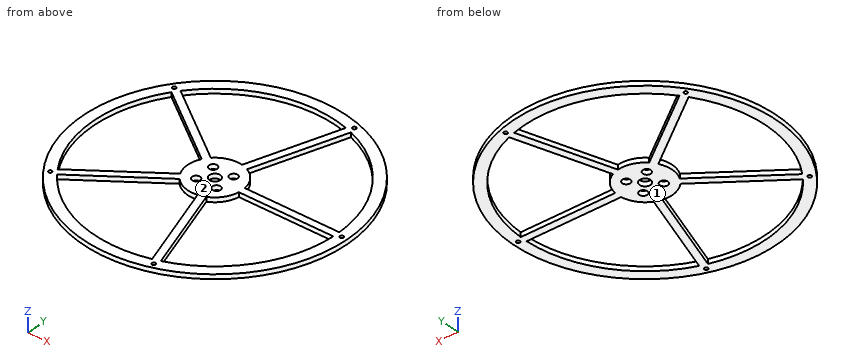
```python
from build123d import *

# Parameters (mm, degrees)
SKETCH_3_R          = 73
EXTRUDE_3_DEPTH     = 2.5
SKETCH_5_R          = 67
CUT_EXTRUDE_1_DEPTH = 2.5
SKETCH_6_R          = 15
EXTRUDE_4_DEPTH     = 2.5
SKETCH_7_R          = 8
CUT_EXTRUDE_2_DEPTH = 2.5
EXTRUDE_6_DEPTH     = 2.5
EXTRUDE_7_DEPTH     = 2.5
EXTRUDE_8_DEPTH     = 2.5
EXTRUDE_9_DEPTH     = 2.5
EXTRUDE_10_DEPTH    = 2.5
SKETCH_14_R         = 8
CUT_EXTRUDE_3_DEPTH = 2.5
SKETCH_15_R         = 1
CUT_EXTRUDE_4_DEPTH = 2.5
SKETCH_16_R         = 8
EXTRUDE_11_DEPTH    = 2.5
SKETCH_17_R         = 3
CUT_EXTRUDE_5_DEPTH = 2.5
SKETCH_18_R         = 3.25
SKETCH_18_R_2       = 2.2
CUT_EXTRUDE_6_DEPTH = 2.5
SKETCH_19_R         = 3.25
EXTRUDE_12_DEPTH    = 2.5
SKETCH_20_R         = 2.2
CUT_EXTRUDE_7_DEPTH = 2.5


with BuildPart() as part:
    # Sketch 3 → Extrude 3 (new body)
    with BuildSketch(Plane.XY):
        Circle(SKETCH_3_R)
    extrude(amount=EXTRUDE_3_DEPTH)

    # Sketch 5 → Cut-Extrude 1 (cut)
    with BuildSketch(Plane.XY.offset(2.5)):
        Circle(SKETCH_5_R)
    extrude(amount=-CUT_EXTRUDE_1_DEPTH, mode=Mode.SUBTRACT)



with BuildPart() as body_2:
    # Sketch 6 → Extrude 4 (new body)
    with BuildSketch(Plane.XY.offset(2.5)):
        Circle(SKETCH_6_R)
    extrude(amount=-EXTRUDE_4_DEPTH)

    # Sketch 7 → Cut-Extrude 2 (cut)
    with BuildSketch(Plane.XY.offset(2.5)):
        Circle(SKETCH_7_R)
    extrude(amount=-CUT_EXTRUDE_2_DEPTH, mode=Mode.SUBTRACT)


with BuildPart() as part_1:
    add(part.part)

    add(body_2.part)  # Extrude 6 merges body 2
    # Sketch 9 → Extrude 6 (add)
    with BuildSketch(Plane.XY.offset(2.5)):
        with BuildLine():
            Line((0, 2), (0, 0))
            Line((0, 0), (0, -2))
            Line((0, -2), (66.970142601, -2))
            ThreePointArc((66.970142601, -2), (67, 0), (66.970142601, 2))
            Line((66.970142601, 2), (0, 2))
        make_face()
    extrude(amount=-EXTRUDE_6_DEPTH)

    # Sketch 10 → Extrude 7 (add)
    with BuildSketch(Plane.XY.offset(2.5)):
        with BuildLine():
            Line((1.902113033, -0.618033989), (0, 0))
            Line((0, 0), (-1.902113033, 0.618033989))
            Line((-1.902113033, 0.618033989), (18.792799147, 64.310424507))
            ThreePointArc((18.792799147, 64.310424507), (20.704138623, 63.720786592), (22.597025212, 63.074356529))
            Line((22.597025212, 63.074356529), (1.902113033, -0.618033989))
        make_face()
    extrude(amount=-EXTRUDE_7_DEPTH)

    # Sketch 11 → Extrude 8 (add)
    with BuildSketch(Plane.XY.offset(2.5)):
        with BuildLine():
            Line((0, 0), (1.175570505, 1.618033989))
            Line((1.175570505, 1.618033989), (-53.004412975, 40.982096154))
            ThreePointArc((-53.004412975, 40.982096154), (-54.204138623, 39.381611904), (-55.355553985, 37.746028176))
            Line((-55.355553985, 37.746028176), (-1.175570505, -1.618033989))
            Line((-1.175570505, -1.618033989), (0, 0))
        make_face()
    extrude(amount=-EXTRUDE_8_DEPTH)

    # Sketch 12 → Extrude 9 (add)
    with BuildSketch(Plane.XY.offset(2.5)):
        with BuildLine():
            Line((0, 0), (1.175570505, -1.618033989))
            Line((1.175570505, -1.618033989), (-53.004412975, -40.982096154))
            ThreePointArc((-53.004412975, -40.982096154), (-54.176759621, -39.419268347), (-55.30304181, -37.822923823))
            Line((-55.30304181, -37.822923823), (-1.175570505, 1.618033989))
            Line((-1.175570505, 1.618033989), (0, 0))
        make_face()
    extrude(amount=-EXTRUDE_9_DEPTH)

    # Sketch 13 → Extrude 10 (add)
    with BuildSketch(Plane.XY.offset(2.5)):
        with BuildLine():
            Line((0, 0), (1.902113033, 0.618033989))
            Line((1.902113033, 0.618033989), (22.597025212, -63.074356529))
            ThreePointArc((22.597025212, -63.074356529), (20.704138623, -63.720786592), (18.792799147, -64.310424507))
            Line((18.792799147, -64.310424507), (-1.902113033, -0.618033989))
            Line((-1.902113033, -0.618033989), (0, 0))
        make_face()
    extrude(amount=-EXTRUDE_10_DEPTH)

    # Sketch 14 → Cut-Extrude 3 (cut)
    with BuildSketch(Plane.XY.offset(2.5)):
        Circle(SKETCH_14_R)
    extrude(amount=-CUT_EXTRUDE_3_DEPTH, mode=Mode.SUBTRACT)

    # Sketch 15 → Cut-Extrude 4 (cut)
    with BuildSketch(Plane.XY.offset(2.5)):
        with Locations((70, 0)):
            Circle(SKETCH_15_R)
        with Locations((21.631189606, 66.573956141)):
            Circle(SKETCH_15_R)
        with Locations((-56.631189606, 41.14496766)):
            Circle(SKETCH_15_R)
        with Locations((-56.631189606, -41.14496766)):
            Circle(SKETCH_15_R)
        with Locations((21.631189606, -66.573956141)):
            Circle(SKETCH_15_R)
    extrude(amount=-CUT_EXTRUDE_4_DEPTH, mode=Mode.SUBTRACT)

    # Sketch 16 → Extrude 11 (add)
    with BuildSketch(Plane.XY.offset(2.5)):
        Circle(SKETCH_16_R)
    extrude(amount=-EXTRUDE_11_DEPTH)

    # Sketch 17 → Cut-Extrude 5 (cut)
    with BuildSketch(Plane.XY.offset(2.5)):
        Circle(SKETCH_17_R)
    extrude(amount=-CUT_EXTRUDE_5_DEPTH, mode=Mode.SUBTRACT)

    # Sketch 18 → Cut-Extrude 6 (cut)
    with BuildSketch(Plane.XY.offset(2.5)):
        with Locations((5.657, 5.657)):
            Circle(SKETCH_18_R)
        with Locations((-5.657, -5.657)):
            Circle(SKETCH_18_R)
        with Locations((5.657, -5.657)):
            Circle(SKETCH_18_R_2)
        with Locations((-5.657, 5.657)):
            Circle(SKETCH_18_R_2)
    extrude(amount=-CUT_EXTRUDE_6_DEPTH, mode=Mode.SUBTRACT)

    # Sketch 19 → Extrude 12 (add)
    with BuildSketch(Plane.XY.offset(2.5)):
        with Locations((5.657, 5.657)):
            Circle(SKETCH_19_R)
        with Locations((-5.657, -5.657)):
            Circle(SKETCH_19_R)
    extrude(amount=-EXTRUDE_12_DEPTH)

    # Sketch 20 → Cut-Extrude 7 (cut)
    with BuildSketch(Plane.XY.offset(2.5)):
        with Locations((5.657, 5.657)):
            Circle(SKETCH_20_R)
        with Locations((-5.657, -5.657)):
            Circle(SKETCH_20_R)
    extrude(amount=-CUT_EXTRUDE_7_DEPTH, mode=Mode.SUBTRACT)


solid = part_1.part
```
Read the model definition and answer for the solid it produces. Units are mm, in the model's axes. Face numbers are marked on the shaded views. Give positions to 0.01 mm unless a question says otherwise; leave off trailing zeros. Write each loop counter-clockwise with the first axis right and the second up, starting at its lowest first coordinate (ties: lowest second). Pieces come first, ordered by that corner, then holes. Notation, with made-up numbers: (1, 34) -> (34, 34) arc R25 ccw to (34, 70) -> close; hole circle Ø3 at (-10.75, 59.25). An arc over 180 degrees is marked (long way). Answer in a Markdown table with one row per item.
1) Determine the mould class of the marked faces 1 and 2 for opening direction Z: released by +Z, released by -Z, zero draft, split by the parting line, or undercut.
Results list:
| item | result |
|---|---|
| face 1 | released by -Z |
| face 2 | released by +Z |
2) Each of these flat-tipped pins is pushed along its axis until it touches: pin 1 Ø1.2 at (x, z) = (42.5, 0.5) entering from -Y; pin 2 Ø1.2 at (x, z) = (28.5, 1.5) entering from +Y; pin 3 Ø1.5 at (y, z) = (-10, 0.5) entering from +X. Where does it stop, or does it pass through?
Results list:
| item | result |
|---|---|
| pin 1 | y = -59.78 |
| pin 2 | y = 67.46 |
| pin 3 | x = 72.41 |
3) Section A-A on x = 0 is taken. Give the vertices of the cut face in (y, z).
Results list:
| item | result |
|---|---|
| outline | (-73, 0) -> (-67, 0) -> (-67, 2.5) -> (-73, 2.5) -> close; (-15, 0) -> (-3, 0) -> (-3, 2.5) -> (-15, 2.5) -> close; (3, 0) -> (15, 0) -> (15, 2.5) -> (3, 2.5) -> close; (67, 0) -> (73, 0) -> (73, 2.5) -> (67, 2.5) -> close |
4) Section C-C on z = 0.8 is taken. Count the separate pieces of the cut face and the enclosed holes in it, plus the area to 3 significant figures.
Results list:
| item | result |
|---|---|
| separate pieces | 1 |
| enclosed holes | 15 |
| area | 4,280 mm^2 |
5) Section D-D on x = -59.5 is taken. Give the vertices of the cut face in (y, z), plus the area to 3 significant figures.
Results list:
| item | result |
|---|---|
| outline | (-42.29, 0) -> (-30.8, 0) -> (-30.8, 2.5) -> (-42.29, 2.5) -> close; (30.8, 0) -> (42.29, 0) -> (42.29, 2.5) -> (30.8, 2.5) -> close |
| area | 57.5 mm^2 |
6) Straight lines are drawn through the part: line 1 (Y direction, x = 0, z = 1.5); line 2 (Y direction, x = 44, z = 1.8); line 3 (X direction, y = 5.5, z = 2.4). For each, find the intervals that lie inside material, in ascending order. Write a range as [from, to].
Results list:
| item | result |
|---|---|
| line 1 | [-73, -67], [-15, -3], [3, 15], [67, 73] |
| line 2 | [-58.25, -50.53], [-2, 2], [50.53, 58.25] |
| line 3 | [-72.79, -66.77], [-13.96, -7.85], [-3.46, 3.46], [7.85, 13.96], [66.77, 72.79] |
7) Section B-B on y = -49 is taken. Give the vertices of the cut face in (x, z).
Results list:
| item | result |
|---|---|
| outline | (-54.11, 0) -> (-45.69, 0) -> (-45.69, 2.5) -> (-54.11, 2.5) -> close; (13.82, 0) -> (18.02, 0) -> (18.02, 2.5) -> (13.82, 2.5) -> close; (45.69, 0) -> (54.11, 0) -> (54.11, 2.5) -> (45.69, 2.5) -> close |
